Autodesk Inventor part; units mm, degrees
ref_plane "YZ Plane" through (0, 0, 0) normal (1, 0, 0) x (0, 1, 0)
ref_plane "XZ Plane" through (0, 0, 0) normal (0, 1, 0) x (-1, 0, 0)
sketch "Sketch1" plane through (0, 0, 0) normal (0, 0, 1) x (1, 0, 0)
  line L0 (0, 6.35) -> (0, 53.34)
  line L1 (0, 53.34) -> (-19.05, 53.34)
  line L2 (-19.05, 53.34) -> (-19.05, 55.245)
  line L3 (-12.7, 48.895) -> (-6.35, 48.895)
  line L4 (-6.35, 48.895) -> (-6.35, 13.335)
  line L5 (-6.35, 13.335) -> (-19.05, 13.335)
  line L6 (-19.05, 13.335) -> (-19.05, 12.7)
  line L7 (-12.7, 8.89) -> (-6.35, 8.89)
  line L8 (-6.35, 8.89) -> (-6.35, 0)
  line L9 (-6.35, 0) -> (0, 0)
  line L10 (-19.05, 55.245) -> (-19.05, 40.005)
  line L11 (-19.05, 40.005) -> (-12.7, 40.005)
  line L12 (-12.7, 40.005) -> (-12.7, 48.895)
  line L13 (-19.05, 12.7) -> (-19.05, 0)
  line L14 (-19.05, 0) -> (-12.7, 0)
  line L15 (-12.7, 0) -> (-12.7, 8.89)
  line L16 (0, 0) -> (0, 6.35)
  line L17 (0, 0) -> (10.16, 0)
  line L18 (10.16, 0) -> (0, 23.7508)
  point P0 (-19.05, 53.34)
  point P1 (-19.05, 11.43)
  dimension "d1" = 35.56
  dimension "d2" = 4.445
  dimension "d3" = 4.445
  dimension "d4" = 6.35
  dimension "d6" = 6.35
  dimension "d7" = 6.35
  dimension "d13" = 13.335
  dimension "d14" = 13.335
  dimension "d35" = 10.16
  dimension "d36" = 66.84
extrude "Extrusion1" add sketch "Sketch1" along normal mid plane 3.81 contours L16 L9 L8 L7 L15 L14 L13 L6 L5 L4 L3 L12 L11 L10 L1 L0
ref_plane "Work Plane1" through (0, 0, 19.685) normal (0, 0, 1) x (1, 0, 0)
mirror "Mirror1" about plane through (0, 0, 19.685) normal (0, 0, 1) of "Extrusion1"
sketch "Sketch4" plane through (0, 0, 19.685) normal (0, 0, 1) x (1, 0, 0)
  line L0 (-6.35, 8.89) -> (-6.35, 0)
  line L1 (-6.35, 0) -> (63.5, 0)
  line L2 (63.5, 0) -> (63.5, 6.35)
  line L3 (63.5, 6.35) -> (-6.35, 6.35)
  line L4 (-6.35, 6.35) -> (-6.35, 0)
  point P0 (0, 0)
  dimension "d23" = 69.85
  dimension "d24" = 6.35
extrude "Extrusion4" add sketch "Sketch4" along normal mid plane 63.5
sketch "Sketch5" plane through (-6.35, 6.35, 51.435) normal (0, 1, 0) x (1, 0, 0)
  line L0 (0, 63.5) -> (69.85, 63.5) construction
  line L1 (69.85, 63.5) -> (69.85, 0) construction
  line L2 (0, 0) -> (69.85, 0) construction
  line L3 (0, 0) -> (0, 63.5) construction
  line L4 (0, 63.5) -> (69.85, 0) construction
  line L5 (69.85, 63.5) -> (0, 0) construction
  circle A0 centre (34.925, 31.75) radius 25.4
  point P0 (6.35, 51.435)
  dimension "d32" = 50.8
fillet "Fillet1" radius 3.175 4 edges at (-6.35, 3.175, 51.435) (63.5, 3.175, 51.435) (63.5, 3.175, -12.065) (-6.35, 3.175, -12.065)
extrude "Extrusion6" cut sketch "Sketch5" against normal through all
sketch "Sketch6" plane through (0, 0, 1.905) normal (0, 0, 1) x (1, 0, 0)
  line L0 (-3.175, 6.35) -> (60.325, 6.35)
  line L1 (10.4354, 6.35) -> (0, 6.35)
  line L2 (10.4354, 6.35) -> (1.4968, 21.8321)
  line L3 (10.4354, 6.35) -> (28.3126, 6.35) construction
  line L4 (1.4968, 21.8321) -> (0, 24.4246)
  line L5 (0, 53.34) -> (0, 6.35)
  line L6 (0, 24.4246) -> (0, 6.35)
  point P0 (0, 0)
  dimension "d37" = 120
extrude "Extrusion7" add sketch "Sketch6" against normal blind 3.81
mirror "Mirror2" about plane through (0, 0, 19.685) normal (0, 0, 1) of "Extrusion7"
fillet "Fillet2" radius 3.175 2 edges at (0, 24.4246, 39.37) (0, 24.4246, 0)
equation "\"d11\" = width"
equation "\"d15\" = oneHalfSpacing"
equation "\"width\" = 3.81"
equation "\"spacing\" = 39.37"
equation "\"oneHalfSpacing\" = 0.5 * spacing"
properties part number "round_2_0_inchHoleV01"
Work out the finished part from the listing and answer in its coordinate system (mm). A direction names the side the tool comes from. Give positions to 0.01 mm unless a question says otherwise; leave off trailing zeros. Loops run counter-clockwise (first coordinate to the right, second up) from the corner with the lowest first, then second, coordinate; pieces in that order, holes last. Notation, with made-up numbers: (51, 30.25) -> (68, 30.25) arc R24 cw to (68, 47.25) -> close; hole circle Ø6 at (-35, 27). An arc over 180 degrees is marked (long way). Put each result on its own line as item: value. Start each with the question number.
Item 1: Each of these flat-tipped pins is pushed along its axis until it touches: P1, Ø1.9, axis at x = -8.5, z = 0.5, coming from the -Y side; P2, Ø1.9, axis at y = 34.5, z = -1, coming from the -X side; P3, Ø1, axis at x = -0.5, z = 2.5, coming from the -Y side; P4, Ø8, axis at x = 27, y = 13.5, coming from the -Z side. Where does it stop, or does it pass through?
Item 2: Which of the six approach directions +Z, -Z, +X, -X, +Y, -Y give full straight-line access (tool end or side, diameter ignored) to faces 1 (the face through (-6.35, 4, 19)), 2 (the face through (44, 0, -2)), 3 (the face through (-13, 13.335, 0))?
Item 3: Find the intervals of material crossed by L1, parallel to X at y = 42.5, z = -1; L2, parallel to Y at x = 0, z = 27; L3, parallel to Z at x = 6, y = 2 (3 decimals), in increasing order. Write a range as [from, to].
Item 4: The mould has two halves that part along Y. Classify faces 4 (the face through (-9, 53.34, 0)), 5 (the face through (-12.7, 4, 0)), 6 (the face through (-12.7, 44, 0)): released by +Y, released by -Y, zero draft, split by the parting line, or undercut.
Item 5: The part is cut by section B-B (z = 13.5). Give the vertices of the cut face in (x, y).
Item 6: The part is cut by section C-C (x = 8). Give the vertices of the cut face in (y, z) (3 decimals), then the cut area to 3 significant figures.
Item 7: The part is cut by section D-D (x = -11). Give the vertices of the cut face in (y, z) (3 decimals), then the cut area to 3 significant figures.
Item 8: The part is cut by section A-A (y = 29). Give the vertices of the cut face in (x, z) (3 decimals), then the cut area to 3 significant figures.
Answers below:
1. P1: y = 8.89
1. P2: x = -6.35
1. P3: y = 0
1. P4: through
2. face 1: +Z, -Z, -Y
2. face 2: +Z, -Z, +X, -X, -Y
2. face 3: +Z, -Z, -X
3. L1: [-19.05, -12.7], [-6.35, 0]
3. L2: [0, 6.35]
3. L3: [-12.065, 8.043], [31.327, 51.435]
4. face 4: released by +Y
4. face 5: zero draft
4. face 6: undercut
5. outline: (-6.35, 0) -> (3.94, 0) -> (3.94, 6.35) -> (-6.35, 6.35) -> close; (53.21, 0) -> (63.5, 0) -> (63.5, 6.35) -> (53.21, 6.35) -> close
6. outline: (0, -12.065) -> (6.35, -12.065) -> (6.35, -1.905) -> (10.568, -1.905) -> (10.568, 1.905) -> (6.35, 1.905) -> (6.35, 4.791) -> (0, 4.791) -> close; (0, 34.579) -> (6.35, 34.579) -> (6.35, 37.465) -> (10.568, 37.465) -> (10.568, 41.275) -> (6.35, 41.275) -> (6.35, 51.435) -> (0, 51.435) -> close
6. area: 246 mm2
7. outline: (8.89, -1.905) -> (13.335, -1.905) -> (13.335, 1.905) -> (8.89, 1.905) -> close; (8.89, 37.465) -> (13.335, 37.465) -> (13.335, 41.275) -> (8.89, 41.275) -> close; (48.895, -1.905) -> (53.34, -1.905) -> (53.34, 1.905) -> (48.895, 1.905) -> close; (48.895, 37.465) -> (53.34, 37.465) -> (53.34, 41.275) -> (48.895, 41.275) -> close
7. area: 67.7 mm2
8. outline: (-6.35, -1.905) -> (0, -1.905) -> (0, 1.905) -> (-6.35, 1.905) -> close; (-6.35, 37.465) -> (0, 37.465) -> (0, 41.275) -> (-6.35, 41.275) -> close
8. area: 48.4 mm2
